Build history of the part. All positions in model axes, mm. Face numbers are marked on the shaded views. Give positions to 0.01 mm unless a question says otherwise; leave off trailing zeros. One line per item, written item: value.
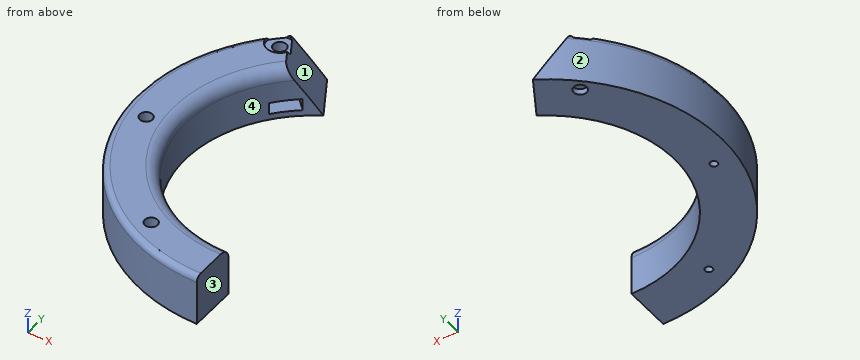
```python
from build123d import *

# Parameters (mm, degrees)
BOSS_EXTRUDE1_DEPTH = 17
SKETCH2_R           = 2.2
CUT_EXTRUDE1_DEPTH  = 86.152803829
CUT_EXTRUDE2_DEPTH  = 86.152803829
DRAFT1_ANGLE        = -32
SKETCH4_R           = 4.5
CUT_EXTRUDE3_DEPTH  = 1.5
FILLET1_R           = 4
CUT_EXTRUDE4_START  = -2
CUT_EXTRUDE4_DEPTH  = 4
SKETCH10_R          = 1.25
CUT_EXTRUDE5_DEPTH  = 86.152803849
SKETCH11_R          = 2.15
CUT_EXTRUDE6_DEPTH  = 14
FILLET2_R           = 2


with BuildPart() as part:
    # Sketch1 → Boss-Extrude1 (new body)
    with BuildSketch(Plane.XY):
        with BuildLine():
            Line((0, 59), (0, 43))
            ThreePointArc((0, 43), (-43, 0), (0, -43))
            Line((0, -43), (0, -59))
            ThreePointArc((0, -59), (-59, 0), (0, 59))
        make_face()
    extrude(amount=BOSS_EXTRUDE1_DEPTH)

    # Sketch2 → Cut-Extrude1 (cut, through all)
    with BuildSketch(Plane.XY.offset(17)):
        with Locations((-38, 40)):
            Circle(SKETCH2_R)
    extrude(amount=-CUT_EXTRUDE1_DEPTH, mode=Mode.SUBTRACT)

    # Sketch3 → Cut-Extrude2 (cut, through all)
    with BuildSketch(Plane.XY.offset(17)):
        Polygon((0, 0), (-48.717134113, 84.380551482), (0, 84.380551482), align=None)
    extrude(amount=-CUT_EXTRUDE2_DEPTH, mode=Mode.SUBTRACT)

    # Draft1
    draft1_faces = [part.faces().sort_by_distance(p)[0] for p in [
        (-25.5, 44.167295593, 8.5),
    ]]
    draft(draft1_faces, Plane(origin=(0, 0, 0), x_dir=(-1, 0, 0), z_dir=(0, 0, -1)), DRAFT1_ANGLE)

    # Sketch4 → Cut-Extrude3 (cut)
    with BuildSketch(Plane.XY.offset(17)):
        with Locations((-38, 40)):
            Circle(SKETCH4_R)
    extrude(amount=-CUT_EXTRUDE3_DEPTH, mode=Mode.SUBTRACT)

    # Fillet1
    fillet1_edges = [part.edges().sort_by_distance(p)[0] for p in [
        (-39.826243941, -16.213275226, 17),
    ]]
    fillet(fillet1_edges, radius=FILLET1_R)

    # Sketch9 → Cut-Extrude4 (cut)
    with BuildSketch(Plane(origin=(0, 0, 0), x_dir=(-1, 0, 0), z_dir=(0, 0, -1)).offset(CUT_EXTRUDE4_START)):
        Polygon((40.91436799, 37.11732892), (41.953650381, 41.082581175), (39.039282391, 43.965252255), (35.08563201, 42.88267108), (21.021032653, 28.663421982), (28.6051551, 21.353976547), align=None)
    extrude(amount=-CUT_EXTRUDE4_DEPTH, mode=Mode.SUBTRACT)

    # Sketch10 → Cut-Extrude5 (cut, through all)
    with BuildSketch(Plane(origin=(0, 0, 0), x_dir=(-1, 0, 0), z_dir=(0, 0, -1))):
        with Locations((24, -46)):
            Circle(SKETCH10_R)
        with Locations((51, -8)):
            Circle(SKETCH10_R)
    extrude(amount=-CUT_EXTRUDE5_DEPTH, mode=Mode.SUBTRACT)

    # Sketch11 → Cut-Extrude6 (cut)
    with BuildSketch(Plane.XY.offset(17)):
        with Locations((-51, -8)):
            Circle(SKETCH11_R)
        with Locations((-24, -46)):
            Circle(SKETCH11_R)
    extrude(amount=-CUT_EXTRUDE6_DEPTH, mode=Mode.SUBTRACT)

    # Fillet2
    # the kernel refuses this fillet: 2 mm, written as the material it takes off along each edge
    with BuildSketch(Plane(origin=(0, 0, 17), x_dir=(-0.7194630608537799, 0.6945307077926146, 0), z_dir=(-0.6945307077926146, -0.7194630608537799, 0))) as fillet2_piece_1:
        with BuildLine():
            CenterArc((59 - FILLET2_R, FILLET2_R), FILLET2_R, 270, 90)
            Line((59 - FILLET2_R, 0), (59, 0))
            Line((59, 0), (59, FILLET2_R))
        make_face()
    revolve(axis=Axis((0, 0, 17), (0, 0, -1)), revolution_arc=10.493238867, mode=Mode.SUBTRACT)
    with BuildSketch(Plane(origin=(0, 0, 17), x_dir=(0.08471968524952049, -0.9964048248233356, 0), z_dir=(0.9964048248233356, 0.08471968524952049, 0))) as fillet2_piece_2:
        with BuildLine():
            CenterArc((59 - FILLET2_R, FILLET2_R), FILLET2_R, 270, 90)
            Line((59, FILLET2_R), (59, 0))
            Line((59, 0), (59 - FILLET2_R, 0))
        make_face()
    revolve(axis=Axis((0, 0, 17), (0, 0, -1)), revolution_arc=143.812006021, mode=Mode.SUBTRACT)


solid = part.part
```
(1) Pull direction Y, two halves, no side cores. Call the marked faces 1, 2, 3 and 4: +Y half, -Y half, draft (parallel to the pull), parting line (faces both ways), or undercut.
Completed:
face 1: +Y half
face 2: parting line
face 3: draft
face 4: undercut
(2) Pin check, flat tips, straight feed: P1, Ø6, axis at x = -12, z = 9.5, coming from the -Y side; P2, Ø4, axis at x = -24, y = -46, coming from the +Z side; P3, Ø1, axis at x = -22.5, z = 8, coming from the -Y side; P4, Ø2.5, axis at x = -38, y = 40, coming from the -Z side. Stop position of each tip, or through.
Completed:
P1: y = -58.31
P2: z = 3
P3: y = -54.74
P4: through
(3) Drill centre lines: line 1 (Y direction, x = -24, z = 0.7); line 2 (Y direction, x = -38, z = 10.25); line 3 (Y direction, x = -50, z = 11.75). Where is each one in solid material? Low to high.
Completed:
line 1: -53.9 to -47.25, -44.75 to -35.68, 35.68 to 40.69
line 2: -45.13 to -20.12, 20.12 to 37.8, 42.2 to 45.13
line 3: -31.32 to -9.9, -6.1 to 31.32
